from build123d import *

# Parameters (mm, degrees)
SKETCH_1_R      = 1
EXTRUDE_1_DEPTH = 4
FILLET_1_R      = 2


with BuildPart() as part:
    # 草图1 → 凸台-拉伸1 (new body)
    with BuildSketch(Plane(origin=(0, 0, 0), x_dir=(1, 0, 0), z_dir=(0, 1, 0))):
        Polygon((22.744681764, 13.741702265), (17.8, 13), (15.217391304, 30.217391304), (25, 40), (30, 45), (30, 65), (36, 65), (36, 43.928932188), (30.292893219, 38.221825407), (20.536171544, 28.465103732), align=None)
        with Locations(Location((33, 52, 0), (0, 0, 270))):
            Circle(SKETCH_1_R, mode=Mode.SUBTRACT)
        with Locations(Location((33, 60, 0), (0, 0, 270))):
            Circle(SKETCH_1_R, mode=Mode.SUBTRACT)
    extrude(amount=EXTRUDE_1_DEPTH)

    # 圆角1
    fillet_1_edges = [part.edges().sort_by_distance(p)[0] for p in [
        (17.8, 2, -13),
        (15.217391304, 2, -30.217391304),
        (30, 2, -45),
        (30, 2, -65),
        (36, 2, -65),
        (36, 2, -43.928932188),
        (20.536171544, 2, -28.465103732),
        (22.744681764, 2, -13.741702265),
    ]]
    fillet(fillet_1_edges, radius=FILLET_1_R)


solid = part.part
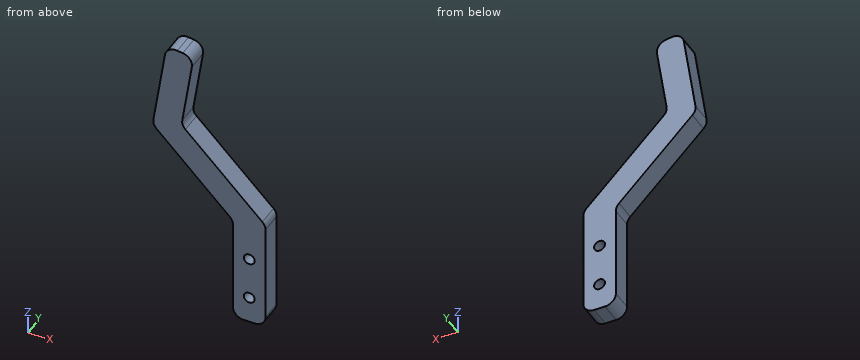
CAD build for the part. Positions are in the model's coordinates, mm. Round coordinates to 2 decimals unless told otherwise and drop trailing zeros. Loops run counter-clockwise (first coordinate to the right, second up) from the corner with the lowest first, then second, coordinate; pieces in that order, holes last.
(1) Cut at C-C (x = 33). Give the cut face in (y, z).
(2) Drop flat-ended pins along their axis: pin 1 (2.5 mm diameter, centred on x = 33, z = -60, fed in from +Y); pin 2 (1.2 mm diameter, centred on y = 2.5, z = -53, fed in from -X). Give the stop position or say it passes through.
(3) Cut at A-A (y = 2.7). Give the cut face in (x, z), plus the area to 3 significant figures.
(4) Cut at B-B (z = -60). Give the cut face in (x, y), plus the area to 3 significant figures.
(5) Wall check: line 1 along Z through (x, y) = (32.5, 1.4); line 2 along X through (y, z) = (2.15, -52); line 3 along X through (y, z) = (2.65, -57). Give the ranges that are in metal, low to high.
(6) Cut at D-D (z = -40). Give the cut face in (x, y), plus the area to 3 significant figures.
Findings below:
1. outline: (0, -65) - (4, -65) - (4, -61) - (0, -61) - close; (0, -59) - (4, -59) - (4, -53) - (0, -53) - close; (0, -51) - (4, -51) - (4, -40.93) - (0, -40.93) - close
2. pin 1: stops at y = 4
2. pin 2: stops at x = 30
3. outline: (15.37, -29.22) arc R2 ccw to (15.93, -30.93) - (29.41, -44.41) arc R2 cw to (30, -45.83) - (30, -63) arc R2 ccw to (32, -65) - (34, -65) arc R2 ccw to (36, -63) - (36, -44.76) arc R2 ccw to (35.41, -43.34) - (21.25, -29.18) arc R2 cw to (20.69, -27.47) - (22.45, -15.72) arc R2 ccw to (20.77, -13.45) - (19.78, -13.3) arc R2 ccw to (17.5, -14.98) - close; hole circle Ø2 at (33, -60); hole circle Ø2 at (33, -52)
3. area: 301 mm2
4. outline: (30, 0) - (32, 0) - (32, 4) - (30, 4) - close; (34, 0) - (36, 0) - (36, 4) - (34, 4) - close
4. area: 16.0 mm2
5. line 1: z = -65 to -60.87, -59.13 to -52.87, -51.13 to -40.43
5. line 2: x = 30 to 32, 34 to 36
5. line 3: x = 30 to 36
6. outline: (25, 0) - (32.07, 0) - (32.07, 4) - (25, 4) - close
6. area: 28.3 mm2
